For this review, take the finished solid that the model builds, in its own axes (mm). Give positions to 0.01 mm unless a question says otherwise; leave off trailing zeros. Order: outer loops, then holes, each group sorted by start corner. A loop starts at its lowest first (then second) coordinate and runs counter-clockwise, first axis right, second up.
Item 1: For P1, Ø2, axis at y = 64, z = 5.5, coming from the +X side; P2, Ø3, axis at y = 87.5, z = 4.5, coming from the -X side; P3, Ø1, axis at x = 16.5, z = 4, coming from the -Y side, all flat-tipped, find the tip position at first contact; note any pin that passes through.
Item 2: Consider section D-D (y = 0). Give the boundary of the cut face in (x, z), plus the area to 3 significant figures.
Item 3: The part is to be moulded in two halves that separate along Y. For faces 1 (the flat face through (-2, -35, 0)), 2 (the cylindrical face through (61.54, 146.337, 3.131)), 3 (the cylindrical face through (-21.855, 166.453, 3.131)), 4 (the cylindrical face through (-14.26, 0.63, 3.13)), say which applies: released by +Y, released by -Y, zero draft, split by the parting line, or undercut.
Item 4: For probe 1 along Y at (x, z) = (-8.5, 5.75); probe 2 along Y at (x, z) = (43.5, 5.75); probe 3 along Y at (x, z) = (3, 3.75), list the stretches that pass through material, from the lowest coordinate up.
Item 5: Consider section A-A (x = 78). Give the boundary of the cut face in (y, z), plus the area to 3 significant figures.
Item 6: Consider section C-C (z = 1.25). Give the boundary of the cut face in (x, y), plus the area to 3 significant figures.
Item 7: Consider section B-B (y = 119). Give the boundary of the cut face in (x, z).
```python
from build123d import *

# Parameters (mm, degrees)
F0_R     = 167.8813
F0_R_2   = 3.373438
F0_R_3   = 14.2748
F1_DEPTH = 6.35


with BuildPart() as f1:
    # F0 (on Top) → F1 (new body)
    with BuildSketch(Plane.XY):
        Circle(F0_R)
        with BuildLine():
            ThreePointArc((158.75, 0), (-112.253202, -112.253201), (1e-06, 158.75))
            ThreePointArc((1e-06, 158.75), (62.366073, 145.986422), (114.703619, 109.748086))
            ThreePointArc((114.703619, 109.748086), (147.327462, 59.128517), (158.75, 0))
        make_face(mode=Mode.SUBTRACT)
        with BuildLine():
            ThreePointArc((-10.511197, 19.845404), (-69.650865, 94.170625), (1e-06, 158.75))
            ThreePointArc((1e-06, 158.75), (-112.253202, -112.253201), (158.75, 0))
            ThreePointArc((158.75, 0), (147.327462, 59.128517), (114.703619, 109.748086))
            ThreePointArc((114.703619, 109.748086), (129.058109, 87.475476), (134.084026, 61.458929))
            ThreePointArc((134.084026, 61.458929), (95.06779, -1.217235), (21.605816, 6.124868))
            ThreePointArc((21.605816, 6.124868), (41.65377, -18.375428), (48.827607, -49.209192))
            ThreePointArc((48.827607, -49.209192), (-73.999887, -94.732897), (-10.511197, 19.845404))
        make_face()
        with Locations((-50.139664, -116.683392)):
            Circle(F0_R_2, mode=Mode.SUBTRACT)
        with Locations((-75.98095, 101.763919)):
            Circle(F0_R_2, mode=Mode.SUBTRACT)
        with Locations((126.120614, 14.919473)):
            Circle(F0_R_2, mode=Mode.SUBTRACT)
        with BuildLine():
            ThreePointArc((21.605816, 6.124868), (6.418678, 15.024834), (-10.511197, 19.845404))
            ThreePointArc((-10.511197, 19.845404), (-73.999887, -94.732897), (48.827607, -49.209192))
            ThreePointArc((48.827607, -49.209192), (41.65377, -18.375428), (21.605816, 6.124868))
        make_face()
        Circle(F0_R_3, mode=Mode.SUBTRACT)
    extrude(amount=F1_DEPTH)


solid = f1.part
```
Resolved:
1. P1: stops at x = 155.61
1. P2: stops at x = -144.18
1. P3: stops at y = -167.12
2. outline: (-167.88, 0) - (-14.27, 0) - (-14.27, 6.35) - (-167.88, 6.35) - close; (14.27, 0) - (31.04, 0) - (31.04, 6.35) - (14.27, 6.35) - close; (97.43, 0) - (167.88, 0) - (167.88, 6.35) - (97.43, 6.35) - close
2. area: 1,530 mm2
3. face 1: zero draft
3. face 2: undercut
3. face 3: split by the parting line
3. face 4: undercut
4. probe 1: y = -167.67 to -11.47, 11.47 to 19.51, 158.23 to 167.67
4. probe 2: y = -162.15 to -5.24, 152.67 to 162.15
4. probe 3: y = -167.85 to -13.96, 13.96 to 16.38, 158.72 to 167.85
5. outline: (-148.66, 0) - (-7.02, 0) - (-7.02, 6.35) - (-148.66, 6.35) - close; (138.27, 0) - (148.66, 0) - (148.66, 6.35) - (138.27, 6.35) - close
5. area: 965 mm2
6. outline: circle Ø335.76 at (0, 0); hole circle Ø6.75 at (-75.98, 101.76); hole circle Ø6.75 at (-50.14, -116.68); hole circle Ø28.55 at (0, 0); hole (-10.51, 19.85) arc R69.85 cw to (21.61, 6.12) arc R69.85 ccw to (134.08, 61.46) arc R69.85 ccw to (114.7, 109.75) arc R158.75 ccw to (0, 158.75) arc R69.85 ccw to start; hole circle Ø6.75 at (126.12, 14.92)
6. area: 62,400 mm2
7. outline: (-118.42, 0) - (-63.03, 0) - (-63.03, 6.35) - (-118.42, 6.35) - close; (105.07, 0) - (118.42, 0) - (118.42, 6.35) - (105.07, 6.35) - close
